Drawing for the job (mm, zero at the part's lowest x, y, z). A direction names the side the tool comes from. Give positions to 0.01 mm unless a question says otherwise; leave off trailing zeros. Order: outer loops, then holes, each group sorted by start corner. A loop starts at its lowest first (then second) coordinate and runs counter-clockwise, first axis right, second up. Notation, with made-up numbers: (18, 7) -> (52, 7) arc R22 ccw to (52, 19) -> close; hole circle Ø7 at (25.5, 37). An arc over 180 degrees is marked (long way). Use one line per item in the form item = value. Start each with the question number.
1) Probe line 1 (X direction, y = 95.5, z = 1.2); line 2 (X direction, y = 9, z = 7). List the from-to ranges inside material, lowest first.
2) Cut at D-D, the plane x = 92. Give the cut face in (y, z).
3) Tool access for the marked faces 1 and 2: list every direction of +Z, -Z, +X, -X, +Y, -Y with a clear straight run to the whole face (end or side of a thin tool).
4) Drop a flat-ended pin along its axis: P1, Ø2.5, axis at x = 67.5, y = 41.5, coming from the +Z side. Give the stop position or say it passes through.
5) Cut at A-A, the plane z = 16.35. Give the cut face in (x, y), and give its area (3 significant figures).
6) Mould opens along X. For the marked faces 3, 4, 5 and 6 say: pulls with the +X half, pulls with the -X half, needs draft (parallel to the pull), parting line crosses it, or undercut.
7) Cut at B-B, the plane y = 50. Give the cut face in (x, z).
8) Cut at C-C, the plane z = 36.5. Give the cut face in (x, y), and give its area (3 significant figures).
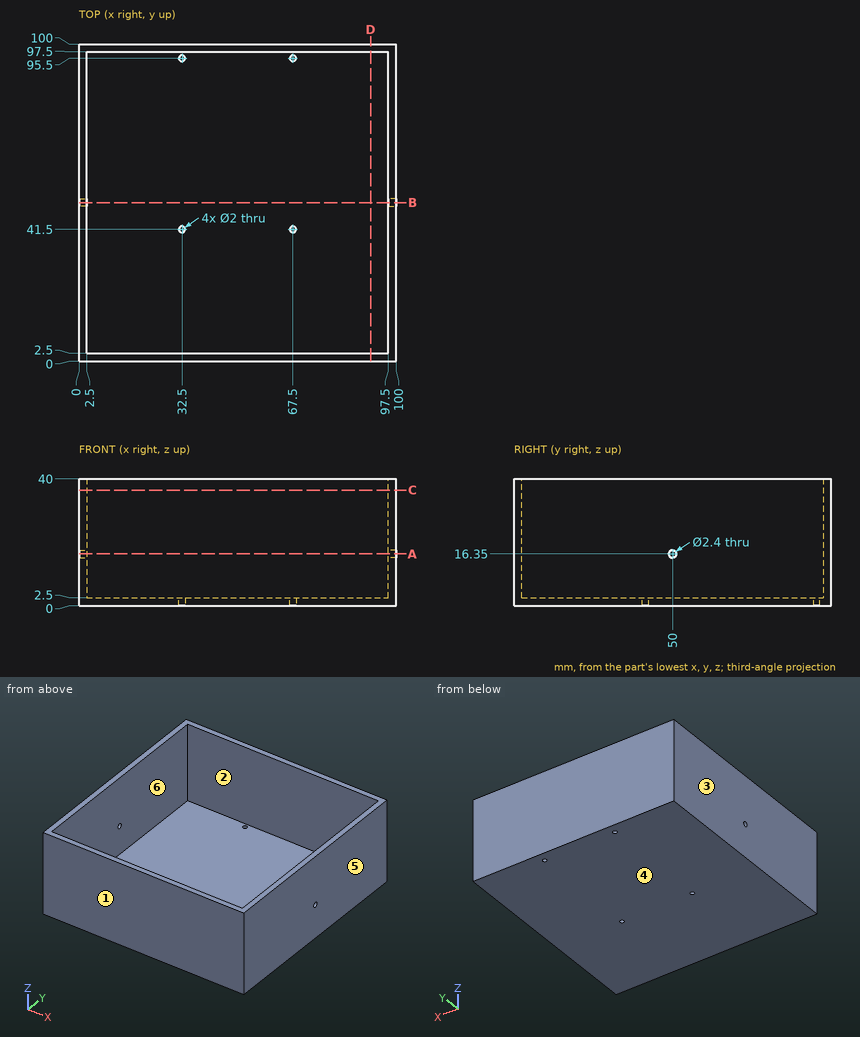
Result:
q1.line_1 = 0 to 31.5, 33.5 to 66.5, 68.5 to 100
q1.line_2 = 0 to 2.5, 97.5 to 100
q2.outline = (0, 0) -> (100, 0) -> (100, 40) -> (97.5, 40) -> (97.5, 2.5) -> (2.5, 2.5) -> (2.5, 40) -> (0, 40) -> close
q3.face_1 = +Z, -Z, +X, -X, -Y
q3.face_2 = +Z
q4.P1 = 2.5
q5.outline = (0, 0) -> (100, 0) -> (100, 48.8) -> (97.5, 48.8) -> (97.5, 2.5) -> (2.5, 2.5) -> (2.5, 48.8) -> (0, 48.8) -> close; (0, 51.2) -> (2.5, 51.2) -> (2.5, 97.5) -> (97.5, 97.5) -> (97.5, 51.2) -> (100, 51.2) -> (100, 100) -> (0, 100) -> close
q5.area = 963 mm²
q6.face_3 = pulls with the -X half
q6.face_4 = needs draft
q6.face_5 = pulls with the +X half
q6.face_6 = undercut
q7.outline = (0, 0) -> (100, 0) -> (100, 15.15) -> (97.5, 15.15) -> (97.5, 2.5) -> (2.5, 2.5) -> (2.5, 15.15) -> (0, 15.15) -> close; (0, 17.55) -> (2.5, 17.55) -> (2.5, 40) -> (0, 40) -> close; (97.5, 17.55) -> (100, 17.55) -> (100, 40) -> (97.5, 40) -> close
q8.outline = (0, 0) -> (100, 0) -> (100, 100) -> (0, 100) -> close; hole (2.5, 2.5) -> (97.5, 2.5) -> (97.5, 97.5) -> (2.5, 97.5) -> close
q8.area = 975 mm²
